Work out the finished part from the listing and answer in its coordinate system (mm). Round coordinates to 2 decimals unless told otherwise and drop trailing zeros. Order: outer loops, then holes, each group sorted by start corner. A loop starts at its lowest first (then second) coordinate and runs counter-clockwise, first axis right, second up. Notation, with made-up numbers: (-14.5, 18.25) -> (-10.5, 18.25) arc R18 ccw to (-10.5, 29.25) -> close; hole circle Ø5 at (-1.75, 24). An arc over 180 degrees is marked (long way). Use a Markdown table: item, result. Add a question column.
Item 1: A cutting plane is placed at C-C, the plane x = 0. Determine the outline of the cut face in (y, z).
Item 2: A cutting plane is placed at D-D, the plane x = 5. Determine the outline of the cut face in (y, z) (3 decimals), plus the area to 4 significant figures.
Item 3: A cutting plane is placed at B-B, the plane y = 0. Determine the outline of the cut face in (x, z) (3 decimals), plus the area to 3 significant figures.
Item 4: A cutting plane is placed at A-A, the plane z = -4. Determine the outline of the cut face in (x, y) (3 decimals), plus the area to 3 significant figures.
Item 5: Find the intervals of material crossed by L1, parallel to X at y = -1.75, z = 4 (3 decimals); L2, parallel to Z at x = 5.25, y = 1.75; L3, parallel to X at y = -2.25, z = 4.25, in increasing order. Write a range as [from, to].
from build123d import *

# Parameters (mm, degrees)
ESQUISSE1_W         = 16
ESQUISSE1_H         = 9
ESQUISSE1_R         = 2
BOSS_EXTRU_1_DEPTH  = 7
TROU_TARAUD_M1_61_D = 1.25
CHANFREIN1_SIZE     = 2
CONG_1_R            = 1


with BuildPart() as part:
    # Esquisse1 → Boss.-Extru.1 (new body)
    with BuildSketch(Plane.XY):
        with Locations((0, 0.5)):
            Rectangle(ESQUISSE1_W, ESQUISSE1_H)
        Circle(ESQUISSE1_R, mode=Mode.SUBTRACT)
    boss_extru_1 = extrude(amount=BOSS_EXTRU_1_DEPTH)

    # Trou taraudé M1.61 (through all)
    with Locations(Plane(origin=(-5, 5, 4), x_dir=(0, 0, 1), z_dir=(0, 1, 0))):
        with Locations((0, 0), (0, 10)):
            trou_taraud_m1_61 = Hole(TROU_TARAUD_M1_61_D / 2)

    # Symétrie1: Boss.-Extru.1, Trou taraudé M1.61 across plane
    add(boss_extru_1.mirror(Plane(origin=(-8, -4, 0), x_dir=(1, 0, 0), z_dir=(0, 0, 1))))
    add(trou_taraud_m1_61.mirror(Plane(origin=(-8, -4, 0), x_dir=(1, 0, 0), z_dir=(0, 0, 1))), mode=Mode.SUBTRACT)

    # Chanfrein1
    chanfrein1_edges = [part.edges().sort_by_distance(p)[0] for p in [
        (8, 0.5, 7),
        (-8, 0.5, 7),
    ]]
    chamfer(chanfrein1_edges, length=CHANFREIN1_SIZE)

    # Congé1
    cong_1_edges = [part.edges().sort_by_distance(p)[0] for p in [
        (-8, 0.5, -7),
        (8, 0.5, -7),
    ]]
    fillet(cong_1_edges, radius=CONG_1_R)


solid = part.part
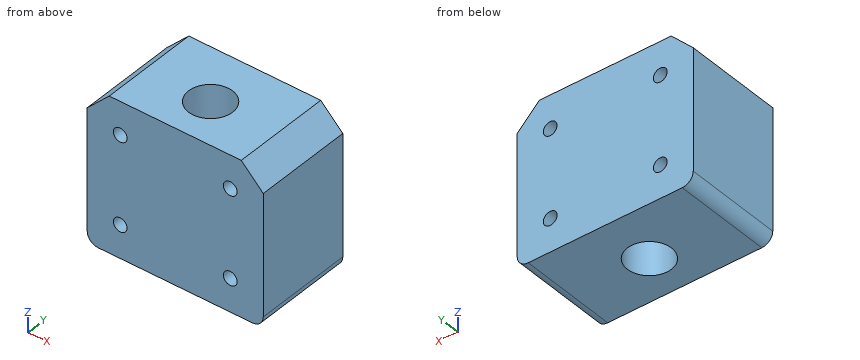
Reported:
| question | item | result |
|---|---|---|
| 1 | outline | (-4, -7) -> (-2, -7) -> (-2, 7) -> (-4, 7) -> close; (2, -7) -> (5, -7) -> (5, 7) -> (2, 7) -> close |
| 2 | outline | (-4, -7) -> (5, -7) -> (5, -4.625) -> (-4, -4.625) -> close; (-4, -3.375) -> (5, -3.375) -> (5, 3.375) -> (-4, 3.375) -> close; (-4, 4.625) -> (5, 4.625) -> (5, 7) -> (-4, 7) -> close |
| 2 | area | 103.5 mm² |
| 3 | outline | (-8, -6) arc R1 ccw to (-7, -7) -> (-2, -7) -> (-2, 7) -> (-6, 7) -> (-8, 5) -> close; (2, -7) -> (7, -7) arc R1 ccw to (8, -6) -> (8, 5) -> (6, 7) -> (2, 7) -> close; hole circle Ø1.25 at (-5, -4); hole circle Ø1.25 at (-5, 4); hole circle Ø1.25 at (5, -4); hole circle Ø1.25 at (5, 4) |
| 3 | area | 159 mm² |
| 4 | outline | (-8, -4) -> (-5.625, -4) -> (-5.625, 5) -> (-8, 5) -> close; (-4.375, -4) -> (4.375, -4) -> (4.375, 5) -> (-4.375, 5) -> close; (5.625, -4) -> (8, -4) -> (8, 5) -> (5.625, 5) -> close; hole circle Ø4 at (0, 0) |
| 4 | area | 109 mm² |
| 5 | L1 | [-8, -5.625], [-4.375, -0.968], [0.968, 4.375], [5.625, 8] |
| 5 | L2 | [-7, -4.57], [-3.43, 3.43], [4.57, 7] |
| 5 | L3 | [-8, -5.57], [-4.43, 4.43], [5.57, 8] |
